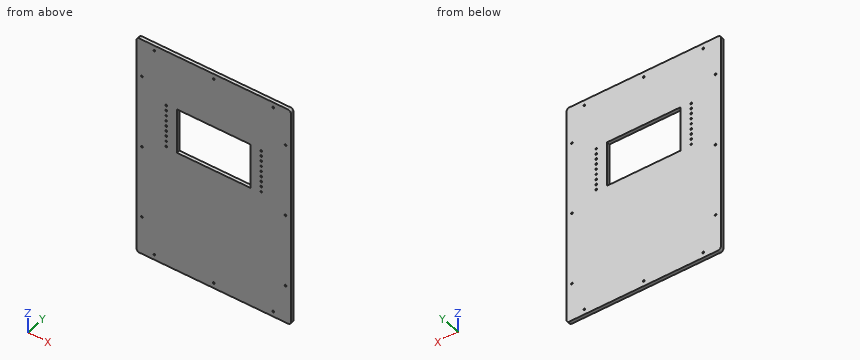
from build123d import *

# Parameters (mm, degrees)
SKETCH1_W                            = 584.2
SKETCH1_H                            = 838.2
LEXAN_BOSS_EXTRUDE1_DEPTH            = 12.7
HOUSING_NEST_HOLE_CUT_EXTRUDE1_REACH = 14.7
SKETCH5_W                            = 280
SKETCH5_H                            = 170
CUT_EXTRUDE7_REACH                   = 14.7
SKETCH6_R                            = 3.25
SKETCH9_R                            = 3.25
CUT_EXTRUDE6_DEPTH                   = 13.7
LPATTERN5_COUNT                      = 5
LPATTERN5_PITCH                      = 20
LPATTERN5_COL_COUNT                  = 5
LPATTERN5_COL_PITCH                  = 20
FILLET3_R                            = 10


with BuildPart() as part:
    # Sketch1 → Lexan Boss-Extrude1 (new body)
    with BuildSketch(Plane(origin=(0, 0, 0), x_dir=(1, 0, 0), z_dir=(0, 1, 0))):
        Rectangle(SKETCH1_W, SKETCH1_H)
    extrude(amount=LEXAN_BOSS_EXTRUDE1_DEPTH)

    # Sketch5 → Housing nest hole Cut-Extrude1 (cut, up to next)
    with BuildSketch(Plane.XZ, mode=Mode.PRIVATE) as housing_nest_hole_cut_extrude1_sk1:
        with Locations((0, 127)):
            Rectangle(SKETCH5_W, SKETCH5_H)
    housing_nest_hole_cut_extrude1_tool1 = extrude(housing_nest_hole_cut_extrude1_sk1.sketch, amount=-HOUSING_NEST_HOLE_CUT_EXTRUDE1_REACH, mode=Mode.PRIVATE) & part.part
    add(housing_nest_hole_cut_extrude1_tool1.solids().sort_by_distance((0, 0, 127))[0], mode=Mode.SUBTRACT)

    # Sketch6 → Cut-Extrude7 (cut, up to next)
    with BuildSketch(Plane.XZ, mode=Mode.PRIVATE) as cut_extrude7_sk1:
        with Locations((-272.1, 275)):
            Circle(SKETCH6_R)
    cut_extrude7_tool1 = extrude(cut_extrude7_sk1.sketch, amount=-CUT_EXTRUDE7_REACH, mode=Mode.PRIVATE) & part.part
    add(cut_extrude7_tool1.solids().sort_by_distance((-272.1, 0, 275))[0], mode=Mode.SUBTRACT)
    # Sketch6 → Cut-Extrude7 (cut, up to next)
    with BuildSketch(Plane.XZ, mode=Mode.PRIVATE) as cut_extrude7_sk2:
        with Locations((-272.1, 0)):
            Circle(SKETCH6_R)
    cut_extrude7_tool2 = extrude(cut_extrude7_sk2.sketch, amount=-CUT_EXTRUDE7_REACH, mode=Mode.PRIVATE) & part.part
    add(cut_extrude7_tool2.solids().sort_by_distance((-272.1, 0, 0))[0], mode=Mode.SUBTRACT)
    # Sketch6 → Cut-Extrude7 (cut, up to next)
    with BuildSketch(Plane.XZ, mode=Mode.PRIVATE) as cut_extrude7_sk3:
        with Locations((-272.1, -275)):
            Circle(SKETCH6_R)
    cut_extrude7_tool3 = extrude(cut_extrude7_sk3.sketch, amount=-CUT_EXTRUDE7_REACH, mode=Mode.PRIVATE) & part.part
    add(cut_extrude7_tool3.solids().sort_by_distance((-272.1, 0, -275))[0], mode=Mode.SUBTRACT)
    # Sketch6 → Cut-Extrude7 (cut, up to next)
    with BuildSketch(Plane.XZ, mode=Mode.PRIVATE) as cut_extrude7_sk4:
        with Locations((272.1, -275)):
            Circle(SKETCH6_R)
    cut_extrude7_tool4 = extrude(cut_extrude7_sk4.sketch, amount=-CUT_EXTRUDE7_REACH, mode=Mode.PRIVATE) & part.part
    add(cut_extrude7_tool4.solids().sort_by_distance((272.1, 0, -275))[0], mode=Mode.SUBTRACT)
    # Sketch6 → Cut-Extrude7 (cut, up to next)
    with BuildSketch(Plane.XZ, mode=Mode.PRIVATE) as cut_extrude7_sk5:
        with Locations((272.1, 0)):
            Circle(SKETCH6_R)
    cut_extrude7_tool5 = extrude(cut_extrude7_sk5.sketch, amount=-CUT_EXTRUDE7_REACH, mode=Mode.PRIVATE) & part.part
    add(cut_extrude7_tool5.solids().sort_by_distance((272.1, 0, 0))[0], mode=Mode.SUBTRACT)
    # Sketch6 → Cut-Extrude7 (cut, up to next)
    with BuildSketch(Plane.XZ, mode=Mode.PRIVATE) as cut_extrude7_sk6:
        with Locations((272.1, 275)):
            Circle(SKETCH6_R)
    cut_extrude7_tool6 = extrude(cut_extrude7_sk6.sketch, amount=-CUT_EXTRUDE7_REACH, mode=Mode.PRIVATE) & part.part
    add(cut_extrude7_tool6.solids().sort_by_distance((272.1, 0, 275))[0], mode=Mode.SUBTRACT)
    # Sketch6 → Cut-Extrude7 (cut, up to next)
    with BuildSketch(Plane.XZ, mode=Mode.PRIVATE) as cut_extrude7_sk7:
        with Locations((-225, 399.1)):
            Circle(SKETCH6_R)
    cut_extrude7_tool7 = extrude(cut_extrude7_sk7.sketch, amount=-CUT_EXTRUDE7_REACH, mode=Mode.PRIVATE) & part.part
    add(cut_extrude7_tool7.solids().sort_by_distance((-225, 0, 399.1))[0], mode=Mode.SUBTRACT)
    # Sketch6 → Cut-Extrude7 (cut, up to next)
    with BuildSketch(Plane.XZ, mode=Mode.PRIVATE) as cut_extrude7_sk8:
        with Locations((0, 399.1)):
            Circle(SKETCH6_R)
    cut_extrude7_tool8 = extrude(cut_extrude7_sk8.sketch, amount=-CUT_EXTRUDE7_REACH, mode=Mode.PRIVATE) & part.part
    add(cut_extrude7_tool8.solids().sort_by_distance((0, 0, 399.1))[0], mode=Mode.SUBTRACT)
    # Sketch6 → Cut-Extrude7 (cut, up to next)
    with BuildSketch(Plane.XZ, mode=Mode.PRIVATE) as cut_extrude7_sk9:
        with Locations((225, 399.1)):
            Circle(SKETCH6_R)
    cut_extrude7_tool9 = extrude(cut_extrude7_sk9.sketch, amount=-CUT_EXTRUDE7_REACH, mode=Mode.PRIVATE) & part.part
    add(cut_extrude7_tool9.solids().sort_by_distance((225, 0, 399.1))[0], mode=Mode.SUBTRACT)
    # Sketch6 → Cut-Extrude7 (cut, up to next)
    with BuildSketch(Plane.XZ, mode=Mode.PRIVATE) as cut_extrude7_sk10:
        with Locations((225, -399.1)):
            Circle(SKETCH6_R)
    cut_extrude7_tool10 = extrude(cut_extrude7_sk10.sketch, amount=-CUT_EXTRUDE7_REACH, mode=Mode.PRIVATE) & part.part
    add(cut_extrude7_tool10.solids().sort_by_distance((225, 0, -399.1))[0], mode=Mode.SUBTRACT)
    # Sketch6 → Cut-Extrude7 (cut, up to next)
    with BuildSketch(Plane.XZ, mode=Mode.PRIVATE) as cut_extrude7_sk11:
        with Locations((0, -399.1)):
            Circle(SKETCH6_R)
    cut_extrude7_tool11 = extrude(cut_extrude7_sk11.sketch, amount=-CUT_EXTRUDE7_REACH, mode=Mode.PRIVATE) & part.part
    add(cut_extrude7_tool11.solids().sort_by_distance((0, 0, -399.1))[0], mode=Mode.SUBTRACT)
    # Sketch6 → Cut-Extrude7 (cut, up to next)
    with BuildSketch(Plane.XZ, mode=Mode.PRIVATE) as cut_extrude7_sk12:
        with Locations((-225, -399.1)):
            Circle(SKETCH6_R)
    cut_extrude7_tool12 = extrude(cut_extrude7_sk12.sketch, amount=-CUT_EXTRUDE7_REACH, mode=Mode.PRIVATE) & part.part
    add(cut_extrude7_tool12.solids().sort_by_distance((-225, 0, -399.1))[0], mode=Mode.SUBTRACT)

    # Sketch9 → Cut-Extrude6 (cut, through all)
    with BuildSketch(Plane(origin=(0, 12.7, 0), x_dir=(1, 0, 0), z_dir=(0, 1, 0))):
        with Locations((-180, -127)):
            Circle(SKETCH9_R)
        with Locations((180, -127)):
            Circle(SKETCH9_R)
    cut_extrude6 = extrude(amount=-CUT_EXTRUDE6_DEPTH, mode=Mode.SUBTRACT)

    # LPattern5: Cut-Extrude6 ×5
    with Locations(*[(0, 0, i * LPATTERN5_PITCH) for i in range(1, LPATTERN5_COUNT)]):
        add(cut_extrude6, mode=Mode.SUBTRACT)

    # LPattern5 col: Cut-Extrude6 ×5
    with Locations(*[(0, 0, -i * LPATTERN5_COL_PITCH) for i in range(1, LPATTERN5_COL_COUNT)]):
        add(cut_extrude6, mode=Mode.SUBTRACT)

    # Fillet3
    fillet3_edges = [part.edges().sort_by_distance(p)[0] for p in [
        (292.1, 6.35, 419.1),
        (-292.1, 6.35, 419.1),
        (-292.1, 6.35, -419.1),
        (292.1, 6.35, -419.1),
    ]]
    fillet(fillet3_edges, radius=FILLET3_R)


solid = part.part
Verification items for the finished model (mm, model axes). Round coordinates to 2 decimals unless told otherwise and drop trailing zeros. Order: outer loops, then holes, each group sorted by start corner. A loop starts at its lowest first (then second) coordinate and runs counter-clockwise, first axis right, second up. Notation, with made-up numbers: (-15.75, -36.5) -> (27.25, -36.5) arc R18 ccw to (27.25, -16.5) -> close; hole circle Ø7 at (57, 55.25). An arc over 180 degrees is marked (long way). Put each result on its own line as item: value.
1) Section check A-A (x = -84.5). Record the cut outline in (y, z).
Final values:
outline: (0, -419.1) -> (12.7, -419.1) -> (12.7, 42) -> (0, 42) -> close; (0, 212) -> (12.7, 212) -> (12.7, 419.1) -> (0, 419.1) -> close
2) Material ranges on line 1 (X direction, y = 5.5, z = 207); line 2 (Z direction, x = 74, y = 1); line 3 (Z direction, x = 272.1, y = 4.75), recorded low to high.
Final values:
line 1: x = -292.1 to -183.25, -176.75 to -140, 140 to 176.75, 183.25 to 292.1
line 2: z = -419.1 to 42, 212 to 419.1
line 3: z = -419.1 to -278.25, -271.75 to -3.25, 3.25 to 271.75, 278.25 to 419.1
3) Section check B-B (y = 8.75). Give the number of separate pieces and of enclosed holes in the cut face, then the cut area to 3 significant figures.
Final values:
separate pieces: 1
enclosed holes: 31
area: 441,000 mm^2
